Autodesk Inventor part; units mm, degrees
ref_plane "YZ Plane" through (0, 0, 0) normal (1, 0, 0) x (0, 1, 0)
ref_plane "XZ Plane" through (0, 0, 0) normal (0, 1, 0) x (-1, 0, 0)
ref_plane "XY Plane" through (0, 0, 0) normal (0, 0, 1) x (1, 0, 0)
sketch "スケッチ1" plane through (0, 0, 0) normal (0, 0, 1) x (1, 0, 0)
  circle A0 centre (0, 0) radius 35
  dimension "d0" = 70
extrude "押し出し1" add sketch "スケッチ1" along normal blind 8.5
sketch "スケッチ2" plane through (0, 0, 8.5) normal (0, 0, 1) x (1, 0, 0)
  circle A0 centre (0, 0) radius 35
  circle A1 centre (0, 0) radius 30
  dimension "d3" = 5
extrude "押し出し2" cut sketch "スケッチ2" against normal blind 6 contours A1
sketch "スケッチ3" plane through (0, 0, 2.5) normal (0, 0, 1) x (1, 0, 0)
  circle A0 centre (0, 0) radius 2
  circle A1 centre (0, 0) radius 9
  dimension "d7" = 4
  dimension "d8" = 18
extrude "押し出し3" add sketch "スケッチ3" along normal blind 5
extrude "押し出し4" cut sketch "スケッチ3" against normal blind 5 contours A0
sketch "スケッチ4" plane through (0, 0, 2.5) normal (0, 0, 1) x (1, 0, 0)
  circle A0 centre (20, 0) radius 7
  circle A1 centre (10, 17.3205) radius 7
  circle A2 centre (-10, 17.3205) radius 7
  circle A3 centre (-20, 0) radius 7
  circle A4 centre (-10, -17.3205) radius 7
  circle A5 centre (10, -17.3205) radius 7
  point P0 (0, 0)
  dimension "d14" = 14
  dimension "d15" = 20
  dimension "d18" = 360
extrude "押し出し5" cut sketch "スケッチ4" against normal blind 5
sketch "スケッチ5" plane through (0, 0, 0) normal (0, 0, -1) x (-1, 0, 0)
  circle A0 centre (0, 0) radius 2
  circle A1 centre (0, 0) radius 30
extrude "押し出し6" cut sketch "スケッチ5" against normal blind 0.1
properties part number "20220524_70アルミホイール"
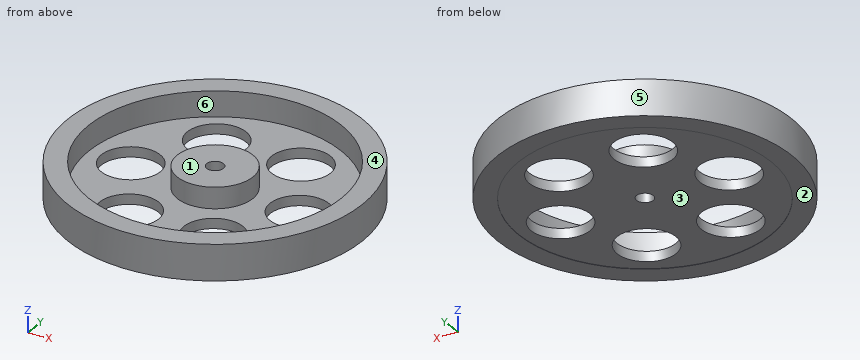
Build history of the part. All positions in model axes, mm. Face numbers are marked on the shaded views. A direction names the side the tool comes from. Coordinates: 2 decimals unless noted, no trailing zeros. Order: outer loops, then holes, each group sorted by start corner. A loop starts at its lowest first (then second) coordinate and runs counter-clockwise, first axis right, second up. Notation, with made-up numbers: (32.5, -0.75) - (59.5, -0.75) arc R17 cw to (59.5, 16.25) - close; hole circle Ø11 at (67.5, -24.5). An arc over 180 degrees is marked (long way). Put each result on its own line as item: value.
1. Probe line 1 along Y through (x, z) = (10, 1.45); line 2 along Y through (x, z) = (0, 4.85); line 3 along Z through (x, y) = (-3, -3). List the from-to ranges inside material, lowest first. Write a range as [from, to].
Answer sheet:
line 1: y = [-33.54, -24.32], [-10.32, 10.32], [24.32, 33.54]
line 2: y = [-35, -30], [-9, -2], [2, 9], [30, 35]
line 3: z = [0.1, 7.5]
2. Pull direction Y, two halves, no side cores. Call the marked faces 4, 5 and 6: pulls with the +Y half, pulls with the -Y half, needs draft (parallel to the pull), parting line crosses it, or undercut.
Answer sheet:
face 4: needs draft
face 5: parting line crosses it
face 6: undercut
3. Saw through at B-B (y = 0). Write the cut outline in (x, z), and give its area (3 significant figures).
Answer sheet:
outline: (-35, 0) - (-30, 0) - (-30, 0.1) - (-27, 0.1) - (-27, 2.5) - (-30, 2.5) - (-30, 8.5) - (-35, 8.5) - close; (-13, 0.1) - (-2, 0.1) - (-2, 7.5) - (-9, 7.5) - (-9, 2.5) - (-13, 2.5) - close; (2, 0.1) - (13, 0.1) - (13, 2.5) - (9, 2.5) - (9, 7.5) - (2, 7.5) - close; (27, 0.1) - (30, 0.1) - (30, 0) - (35, 0) - (35, 8.5) - (30, 8.5) - (30, 2.5) - (27, 2.5) - close
area: 222 mm^2
4. Drop flat-ended pins along their axis: P1, Ø3, axis at y = -16.5, z = 3.5, coming from the -X side; P2, Ø1, axis at x = -9.5, z = 3, coming from the +Y side; P3, Ø1, axis at x = -27.5, z = 7, coming from the +Y side. Give the stop position or say it passes through.
Answer sheet:
P1: stops at x = -31.62
P2: stops at y = 33.82
P3: stops at y = 22.27
5. Saw through at C-C (y = 12). Write the cut outline in (x, z).
Answer sheet:
outline: (-32.88, 0) - (-27.5, 0) - (-27.5, 0.1) - (-14.55, 0.1) - (-14.55, 2.5) - (-27.5, 2.5) - (-27.5, 8.5) - (-32.88, 8.5) - close; (-5.45, 0.1) - (5.45, 0.1) - (5.45, 2.5) - (-5.45, 2.5) - close; (14.55, 0.1) - (27.5, 0.1) - (27.5, 0) - (32.88, 0) - (32.88, 8.5) - (27.5, 8.5) - (27.5, 2.5) - (14.55, 2.5) - close
6. Tool access for the marked faces 1, 2 and 3: list every direction of +Z, -Z, +X, -X, +Y, -Y with a clear straight run to the whole face (end or side of a thin tool).
Answer sheet:
face 1: +Z
face 2: -Z, +X, -X, +Y, -Y
face 3: -Z
7. Saw through at D-D (z = 4.5). Write the cut outline in (x, y).
Answer sheet:
outline: circle Ø70 at (0, 0); circle Ø18 at (0, 0); hole circle Ø60 at (0, 0); hole circle Ø4 at (0, 0)
8. Saw through at A-A (x = 0). Write the cut outline in (y, z).
Answer sheet:
outline: (-35, 0) - (-30, 0) - (-30, 0.1) - (-2, 0.1) - (-2, 7.5) - (-9, 7.5) - (-9, 2.5) - (-30, 2.5) - (-30, 8.5) - (-35, 8.5) - close; (2, 0.1) - (30, 0.1) - (30, 0) - (35, 0) - (35, 8.5) - (30, 8.5) - (30, 2.5) - (9, 2.5) - (9, 7.5) - (2, 7.5) - close
